from build123d import *

# Parameters (mm, degrees)
F0_R     = 3.302
F1_DEPTH = 12.7


with BuildPart() as f1:
    # F0 (on Front) → F1 (new body)
    with BuildSketch(Plane.XZ):
        with BuildLine():
            ThreePointArc((-25.4, 0), (0, -25.4), (25.4, 0))
            ThreePointArc((25.4, 0), (17.960512, 17.960512), (0, 25.4))
            ThreePointArc((0, 25.4), (-17.960512, 17.960512), (-25.4, 0))
        make_face()
        Circle(F0_R, mode=Mode.SUBTRACT)
        with BuildLine():
            ThreePointArc((-25.4, 0), (-17.960512, 17.960512), (0, 25.4))
            Line((0, 25.4), (0, 43.026961))
            ThreePointArc((0, 43.026961), (-18.83358, 25.134302), (-25.4, 0))
        make_face()
    extrude(amount=F1_DEPTH)


solid = f1.part
The model under review builds one solid part; all positions refer to its coordinate system, in mm. A direction names the side the tool comes from. Coordinates: 2 decimals unless noted, no trailing zeros. Write each loop counter-clockwise with the first axis right and the second up, starting at its lowest first coordinate (ties: lowest second). Pieces come first, ordered by that corner, then holes. Notation, with made-up numbers: M 50.5,-22.5 L 103.5,-22.5 A23 ccw 103.5,-9.5 Z; hole C -2,-38 d8. An arc over 180 degrees is marked long. Put each result on its own line as item: value.
1) Add section A-A on y = -1.25. Give the boundary of the cut face in (x, z).
Computed:
outline: M -25.4,0 A25.4 ccw long 0,25.4 L 0,43.03 A47.37 ccw Z; hole C 0,0 d6.6
2) Add section B-B on z = -7. Give the boundary of the cut face in (x, y), then the cut area to 3 significant figures.
Computed:
outline: M -24.42,-12.7 L 24.42,-12.7 L 24.42,0 L -24.42,0 Z
area: 620 mm2
3) Wall thickness on probe 1 along Z at (x, y) = (1, -4.5); probe 2 along X at (y, z) = (-10.5, 1); probe 3 along X at (y, z) = (-4, 3): over which ranges is each line inside the solid? List them lowest first. Write a range as [from, to].
Computed:
probe 1: z = [-25.38, -3.15], [3.15, 25.38]
probe 2: x = [-25.41, -3.15], [3.15, 25.38]
probe 3: x = [-25.37, -1.38], [1.38, 25.22]
4) For faces 1 (the flat face through (0, -6, 34)), 2 (the flat face through (0, 0, 9)), list the 3-axis set-ups (+Z, -Z, +X, -X, +Y, -Y) from which the entire face can be reached by the end or side of a thin tool; tool diameter is ignored.
Computed:
face 1: +Z, +X, +Y, -Y
face 2: +Z, -Z, +X, -X, +Y
5) Add section C-C on x = -13. Give the boundary of the cut face in (y, z).
Computed:
outline: M -12.7,-21.82 L 0,-21.82 L 0,33.02 L -12.7,33.02 Z
6) Clearance check with flat-ended pins moving along their axes: pin 1 Ø1.5 at (y, z) = (-7, 32.5) entering from +X; pin 2 Ø4 at (y, z) = (-4.5, 6.5) entering from -X; pin 3 Ø1.5 at (x, y) = (6, -5.5) entering from -Z. State where each tip first meets the part, or that it passes through.
Computed:
pin 1: stops at x = 0
pin 2: stops at x = -25.29
pin 3: stops at z = -24.85
